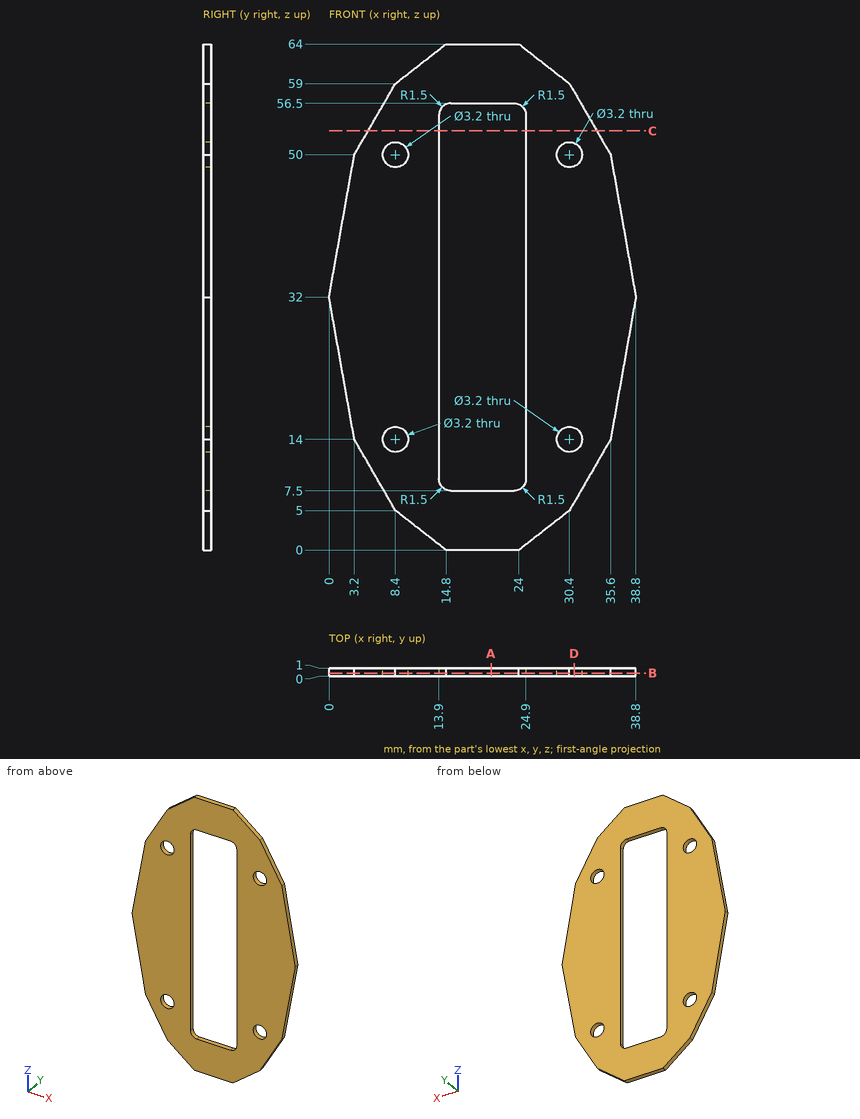
Input: dimensioned drawing with shaded views. Units: mm. Origin: part minimum x, y, z. Coordinates: 2 decimals unless noted, no trailing zeros. Order: outer loops, then holes, each group sorted by start corner. A loop starts at its lowest first (then second) coordinate and runs counter-clockwise, first axis right, second up.
Item 1: Section query A-A (x = 20.5). Output: boundary loops of the cut face in (y, z), then the cut area to 3 significant figures.
Answer:
outline: (0, 0) - (1, 0) - (1, 7.5) - (0, 7.5) - close; (0, 56.5) - (1, 56.5) - (1, 64) - (0, 64) - close
area: 15.0 mm2
Item 2: Section query C-C (z = 53). Output: boundary loops of the cut face in (x, y), then the cut area to 3 significant figures.
Answer:
outline: (4.93, 0) - (13.9, 0) - (13.9, 1) - (4.93, 1) - close; (24.9, 0) - (33.87, 0) - (33.87, 1) - (24.9, 1) - close
area: 17.9 mm2
Item 3: Material intervals for line 1 along X through (y, z) = (0.9, 14); line 2 along Z through (x, y) = (21.5, 0.95); line 3 along X through (y, z) = (0.45, 46), sorted ascending.
Answer:
line 1: x = 3.2 to 6.8, 10 to 13.9, 24.9 to 28.8, 32 to 35.6
line 2: z = 0 to 7.5, 56.5 to 64
line 3: x = 2.49 to 13.9, 24.9 to 36.31
Item 4: Section query D-D (x = 31). Output: boundary loops of the cut face in (y, z), then the cut area to 3 significant figures.
Answer:
outline: (0, 6.04) - (1, 6.04) - (1, 12.52) - (0, 12.52) - close; (0, 15.48) - (1, 15.48) - (1, 48.52) - (0, 48.52) - close; (0, 51.48) - (1, 51.48) - (1, 57.96) - (0, 57.96) - close
area: 46.0 mm2
Item 5: Contact query for flat-ended pins moving along their axis: P1, Ø5, axis at x = 30.4, z = 14, coming from the +Y side; P2, Ø5, axis at x = 17.5, z = 34.5, coming from the -Y side. Output: stop coordinate, or through.
Answer:
P1: stops at y = 1
P2: passes through
Item 6: Section query B-B (y = 0.35). Output: boundary loops of the cut face in (x, z), then the cut area to 3 significant figures.
Answer:
outline: (0, 32) - (3.2, 14) - (8.4, 5) - (14.8, 0) - (24, 0) - (30.4, 5) - (35.6, 14) - (38.8, 32) - (35.6, 50) - (30.4, 59) - (24, 64) - (14.8, 64) - (8.4, 59) - (3.2, 50) - close; hole circle Ø3.2 at (8.4, 14); hole circle Ø3.2 at (8.4, 50); hole (13.9, 9) arc R1.5 ccw to (15.4, 7.5) - (23.4, 7.5) arc R1.5 ccw to (24.9, 9) - (24.9, 55) arc R1.5 ccw to (23.4, 56.5) - (15.4, 56.5) arc R1.5 ccw to (13.9, 55) - close; hole circle Ø3.2 at (30.4, 14); hole circle Ø3.2 at (30.4, 50)
area: 1,360 mm2
